```python
from build123d import *

# Parameters (mm, degrees)
SKETCH1_W             = 217
SKETCH1_H             = 229
BOSS_EXTRUDE1_DEPTH   = 25
EXTRUDE_THIN1_START   = -25
EXTRUDE_THIN1_DEPTH   = 95
FILLET1_R             = 10
CUT_EXTRUDE1_DEPTH    = 20
BOSS_EXTRUDE3_START   = 10
SKETCH10_R            = 38.166666667
BOSS_EXTRUDE3_DEPTH   = 119
SKETCH11_R            = 17
CUT_EXTRUDE2_DEPTH    = 119
BOSS_EXTRUDE4_START   = 10
SKETCH12_R            = 43.666666667
BOSS_EXTRUDE4_DEPTH   = 119
SKETCH13_R            = 17
CUT_EXTRUDE3_DEPTH    = 119
CHAMFER1_SIZE         = 2
CHAMFER1_SIZE2        = 1.154700538
CHAMFER1_PART_2_SIZE  = 2
CHAMFER1_PART_2_SIZE2 = 1.154700538
CHAMFER1_PART_3_SIZE  = 2
CHAMFER1_PART_3_SIZE2 = 1.154700538
CHAMFER1_PART_4_SIZE  = 2
CHAMFER1_PART_4_SIZE2 = 1.154700538
CUT_EXTRUDE4_DEPTH    = 20
CUT_EXTRUDE5_START    = -30
SKETCH16_R            = 38.166666667
SKETCH16_R_2          = 28.166666667
CUT_EXTRUDE5_DEPTH    = 30
BOSS_EXTRUDE5_REACH   = 115.667
SKETCH17_W            = 15
SKETCH17_H            = 30


with BuildPart() as part:
    # Sketch1 → Boss-Extrude1 (new body)
    with BuildSketch(Plane(origin=(0, 0, 0), x_dir=(1, 0, 0), z_dir=(0, 1, 0))):
        with Locations((-108.5, 114.5)):
            Rectangle(SKETCH1_W, SKETCH1_H)
    extrude(amount=BOSS_EXTRUDE1_DEPTH)

    # Sketch2 → Extrude-Thin1 (add)
    with BuildSketch(Plane(origin=(0, 25, 0), x_dir=(1, 0, 0), z_dir=(0, 1, 0)).offset(EXTRUDE_THIN1_START)):
        with BuildLine():
            Line((-163, 0), (-163, 80))
            ThreePointArc((-163, 80), (-104.310137162, 104.310137162), (-80, 163))
            Line((-80, 163), (0, 163))
            Line((0, 163), (0, 148))
            Line((0, 148), (-66.154762636, 148))
            ThreePointArc((-66.154762636, 148), (-93.703535444, 93.703535444), (-148, 66.154762636))
            Line((-148, 66.154762636), (-148, 0))
            Line((-148, 0), (-163, 0))
        make_face()
    extrude(amount=EXTRUDE_THIN1_DEPTH)

    # Fillet1
    fillet1_edges = [part.edges().sort_by_distance(p)[0] for p in [
        (0, 12.5, 0),
        (-217, 12.5, 0),
        (-217, 12.5, -229),
        (0, 12.5, -229),
    ]]
    fillet(fillet1_edges, radius=FILLET1_R)

    # Sketch9 → Cut-Extrude1 (cut)
    with BuildSketch(Plane(origin=(0, 25, 0), x_dir=(1, 0, 0), z_dir=(0, 1, 0))):
        with BuildLine():
            Line((-129, 9), (-19, 9))
            ThreePointArc((-19, 9), (-11.928932188, 11.928932188), (-9, 19))
            Line((-9, 19), (-9, 129))
            ThreePointArc((-9, 129), (-11.928932188, 136.071067812), (-19, 139))
            Line((-19, 139), (-51.049117913, 139))
            ThreePointArc((-51.049117913, 139), (-57.004794657, 137.033051383), (-60.617569374, 131.905982906))
            ThreePointArc((-60.617569374, 131.905982906), (-87.339574413, 87.339574413), (-131.905982906, 60.617569374))
            ThreePointArc((-131.905982906, 60.617569374), (-137.033051383, 57.004794657), (-139, 51.049117913))
            Line((-139, 51.049117913), (-139, 19))
            ThreePointArc((-139, 19), (-136.071067812, 11.928932188), (-129, 9))
        make_face()
    extrude(amount=-CUT_EXTRUDE1_DEPTH, mode=Mode.SUBTRACT)

    # Sketch10 → Boss-Extrude3 (add)
    with BuildSketch(Plane.XY.offset(BOSS_EXTRUDE3_START)):
        with Locations((-155.5, 95)):
            Circle(SKETCH10_R)
    extrude(amount=-BOSS_EXTRUDE3_DEPTH)

    # Sketch11 → Cut-Extrude2 (cut)
    with BuildSketch(Plane.XY.offset(10)):
        with Locations((-155.5, 95)):
            Circle(SKETCH11_R)
    extrude(amount=-CUT_EXTRUDE2_DEPTH, mode=Mode.SUBTRACT)

    # Sketch12 → Boss-Extrude4 (add)
    with BuildSketch(Plane(origin=(0, 0, 0), x_dir=(0, 0, -1), z_dir=(1, 0, 0)).offset(BOSS_EXTRUDE4_START)):
        with Locations((155.5, 95)):
            Circle(SKETCH12_R)
    extrude(amount=-BOSS_EXTRUDE4_DEPTH)

    # Sketch13 → Cut-Extrude3 (cut)
    with BuildSketch(Plane(origin=(10, 0, 0), x_dir=(0, 0, -1), z_dir=(1, 0, 0))):
        with Locations((155.5, 95)):
            Circle(SKETCH13_R)
    extrude(amount=-CUT_EXTRUDE3_DEPTH, mode=Mode.SUBTRACT)

    # Chamfer1
    chamfer1_edges = [part.edges().sort_by_distance(p)[0] for p in [
        (-172.5, 95, 10),
    ]]
    chamfer1_side = [part.faces().sort_by_distance(p)[0] for p in [
        (-192.587150314, 95, 10),
    ]]
    chamfer(chamfer1_edges, length=CHAMFER1_SIZE, length2=CHAMFER1_SIZE2, reference=chamfer1_side[0])

    # Chamfer1 part 2
    chamfer1_part_2_edges = [part.edges().sort_by_distance(p)[0] for p in [
        (-172.5, 95, -109),
    ]]
    chamfer1_part_2_side = [part.faces().sort_by_distance(p)[0] for p in [
        (-192.587150314, 95, -109),
    ]]
    chamfer(chamfer1_part_2_edges, length=CHAMFER1_PART_2_SIZE, length2=CHAMFER1_PART_2_SIZE2, reference=chamfer1_part_2_side[0])

    # Chamfer1 part 3
    chamfer1_part_3_edges = [part.edges().sort_by_distance(p)[0] for p in [
        (10, 95, -138.5),
    ]]
    chamfer1_part_3_side = [part.faces().sort_by_distance(p)[0] for p in [
        (10, 95, -113.068413178),
    ]]
    chamfer(chamfer1_part_3_edges, length=CHAMFER1_PART_3_SIZE, length2=CHAMFER1_PART_3_SIZE2, reference=chamfer1_part_3_side[0])

    # Chamfer1 part 4
    chamfer1_part_4_edges = [part.edges().sort_by_distance(p)[0] for p in [
        (-109, 95, -138.5),
    ]]
    chamfer1_part_4_side = [part.faces().sort_by_distance(p)[0] for p in [
        (-109, 95, -113.068413178),
    ]]
    chamfer(chamfer1_part_4_edges, length=CHAMFER1_PART_4_SIZE, length2=CHAMFER1_PART_4_SIZE2, reference=chamfer1_part_4_side[0])

    # Sketch15 → Cut-Extrude4 (cut)
    with BuildSketch(Plane(origin=(0, 25, 0), x_dir=(1, 0, 0), z_dir=(0, 1, 0))):
        with BuildLine():
            Line((-89, 163), (-89, 210))
            ThreePointArc((-89, 210), (-91.928932188, 217.071067812), (-99, 220))
            Line((-99, 220), (-198, 220))
            ThreePointArc((-198, 220), (-205.071067812, 217.071067812), (-208, 210))
            Line((-208, 210), (-208, 99))
            ThreePointArc((-208, 99), (-205.071067812, 91.928932188), (-198, 89))
            Line((-198, 89), (-163, 89))
            ThreePointArc((-163, 89), (-110.674098192, 110.674098192), (-89, 163))
        make_face()
    extrude(amount=-CUT_EXTRUDE4_DEPTH, mode=Mode.SUBTRACT)

    # Sketch16 → Cut-Extrude5 (cut)
    with BuildSketch(Plane.XY.offset(10).offset(CUT_EXTRUDE5_START)):
        with Locations((-155.5, 95)):
            Circle(SKETCH16_R)
        with Locations((-155.5, 95)):
            Circle(SKETCH16_R_2, mode=Mode.SUBTRACT)
    extrude(amount=-CUT_EXTRUDE5_DEPTH, mode=Mode.SUBTRACT)

    # Sketch17 → Boss-Extrude5 (add, up to next)
    with BuildSketch(Plane(origin=(0, 25, 0), x_dir=(1, 0, 0), z_dir=(0, 1, 0)), mode=Mode.PRIVATE) as boss_extrude5_sk1:
        with Locations((-155.5, 35)):
            Rectangle(SKETCH17_W, SKETCH17_H)
    boss_extrude5_tool1 = extrude(boss_extrude5_sk1.sketch, amount=BOSS_EXTRUDE5_REACH, mode=Mode.PRIVATE) - part.part
    add(boss_extrude5_tool1.solids().sort_by_distance((-155.5, 25, -35))[0])


solid = part.part
```
Geometry check sheet. Reference: the model listing, model coordinates, mm. A direction names the side the tool comes from. Coordinates: 2 decimals unless noted, no trailing zeros. Write each loop counter-clockwise with the first axis right and the second up, starting at its lowest first coordinate (ties: lowest second). Pieces come first, ordered by that corner, then holes. Notation, with made-up numbers: (39, 67.25) -> (93, 67.25) arc R26 cw to (93, 106.25) -> close; hole circle Ø2 at (-4, 10). An arc over 180 degrees is marked (long way). Use CSV: the item, a comma, the result in double quotes. Start each with the question number.
Item 1: Set-up check for faces 4 (the cylindrical face through (-193.63, 96.68, -4.79)), 5 (the flat face through (-148, 15, -220)), 6 (the flat face through (-91, 25, -85)), 7 (the flat face through (-149, 5, -155)): record each of +Z, -Z, +X, -X, +Y, -Y from which the full face is reachable in a straight line by a thin tool's end or side.
Item 2: Cross-section at A-A, the plane x = -28. Record the cut outline in (y, z), plus the area to 3 significant figures.
Item 3: Cross-section at D-D, the plane z = -190. Record the cut outline in (x, y), plus the area to 3 significant figures.
Item 4: Mould release check, pull along Y, two halves, no side actions. Record for faces 1 (the cylindrical face through (-12.01, 15.14, -11.85)), 2 (the flat face through (-107, 0, -116)), 3 (the cylindrical face through (-86.82, 15.14, -87.86)): released by +Y, released by -Y, zero draft, split by the parting line, or undercut.
Item 5: Depth check by flat-ended pin: pin 1 Ø5 at (x, y) = (-164.5, 67) entering from -Z; pin 2 Ø8 at (x, z) = (-127.5, -172.5) entering from +Y; pin 3 Ø4 at (x, y) = (-71, 60.5) entering from -Z. Enter the tip coordinate at first touch or a pass-through.
Item 6: Cross-section at C-C, the plane y = 13. Record the cut outline in (x, z), plus the area to 3 significant figures.
Item 7: Cross-section at B-B, the plane z = -47. Record the cut outline in (x, y), plus the area to 3 significant figures.
Item 8: Thickness scan on line 1 (Y direction, x = -155.5, z = -38); line 2 (X direction, y = 10.5, z = -110); line 3 (Y direction, x = -143.5, z = -50.5). Record the ranges inside material, lowest first.
Answers:
1,face 4,"+Z"
1,face 5,"+Y"
1,face 6,"+Z, +X"
1,face 7,"none"
2,outline,"(0, -229) -> (25, -229) -> (25, -163) -> (51.98, -163) arc R43.67 ccw (long way) to (51.98, -148) -> (25, -148) -> (25, -139) -> (5, -139) -> (5, -9) -> (25, -9) -> (25, 0) -> (0, 0) -> close; hole circle Ø34 at (95, -155.5)"
2,area,"8,610 mm^2"
3,outline,"(-217, 0) -> (0, 0) -> (0, 25) -> (-89, 25) -> (-89, 5) -> (-208, 5) -> (-208, 25) -> (-217, 25) -> close; (-109, 68.23) -> (10, 68.23) -> (10, 121.77) -> (-109, 121.77) -> close"
3,area,"9,420 mm^2"
4,face 1,"zero draft"
4,face 2,"released by -Y"
4,face 3,"undercut"
5,pin 1,"z = -109"
5,pin 2,"y = 5"
5,pin 3,"z = -184.66"
6,outline,"(-217, -219) arc R10 ccw to (-207, -229) -> (-10, -229) arc R10 ccw to (0, -219) -> (0, -10) arc R10 ccw to (-10, 0) -> (-207, 0) arc R10 ccw to (-217, -10) -> close; hole (-208, -210) arc R10 ccw to (-198, -220) -> (-99, -220) arc R10 ccw to (-89, -210) -> (-89, -163) arc R74 ccw to (-163, -89) -> (-198, -89) arc R10 ccw to (-208, -99) -> close; hole (-139, -51.05) arc R10 ccw to (-131.91, -60.62) arc R107 cw to (-60.62, -131.91) arc R10 ccw to (-51.05, -139) -> (-19, -139) arc R10 ccw to (-9, -129) -> (-9, -19) arc R10 ccw to (-19, -9) -> (-129, -9) arc R10 ccw to (-139, -19) -> close"
6,area,"22,900 mm^2"
7,outline,"(-217, 0) -> (0, 0) -> (0, 25) -> (-9, 25) -> (-9, 5) -> (-139, 5) -> (-139, 25) -> (-148, 25) -> (-148, 67.85) arc R28.17 ccw (long way) to (-163, 67.85) -> (-163, 25) -> (-217, 25) -> close; hole circle Ø34 at (-155.5, 95)"
7,area,"5,040 mm^2"
8,line 1,"0 to 78, 112 to 123.17"
8,line 2,"-217 to -208, -111.36 to -70.05, -9 to 0"
8,line 3,"0 to 25, 58.77 to 82.96, 107.04 to 131.23"
